The model under review builds one solid part; all positions refer to its coordinate system, in mm. A direction names the side the tool comes from. Round coordinates to 2 decimals unless told otherwise and drop trailing zeros. Order: outer loops, then holes, each group sorted by start corner. A loop starts at its lowest first (then second) coordinate and runs counter-clockwise, first axis right, second up. Notation, with made-up numbers: M 25,-5.5 L 41,-5.5 A9 cw 41,5.5 Z; hole C -28.75,6.5 d10. An arc over 180 degrees is marked long. Answer as a JSON object with one key per item and string values. Group by question number.
1. Mouldability with a two-part tool opening along X and no side actions: class faces 1 (the face through (454.06, -0.04, 521.2)), 2 (the face through (914.4, 0, 1002)), 3 (the face through (0, 0, 1002)), 4 (the face through (451, 0, 0)) as released by +X, released by -X, zero draft, split by the parting line, or undercut.
2. Add section B-B on z = 642. State the section outline as (x, y) points (3 decimals).
3. To check wall thickness, follow probe 1 along Z at (x, y) = (260.5, -4); probe 2 along X at (y, z) = (9, 579); probe 3 along Z at (x, y) = (315, 10) (1 decimal). State the ranges of each line that lie inside material, in increasing order. Write a range as [from, to].
4. Clearance check with flat-ended pins moving along their axes: P1, Ø3, axis at y = -12.5, z = 993, coming from the -X side; P2, Ø4, axis at x = 579, z = 665.5, coming from the -Y side (3 decimals); P3, Ø6, axis at x = 260, z = 1415, coming from the +Y side (3 decimals). State where each tip first meets the part, or that it passes through.
5. Machinability: for faces 5 (the face through (453, 3.175, 1441)), 6 (the face through (44, -22.225, 1030)), 7 (the face through (460.344, -0.044, 518.616)), 8 (the face through (453, -3.175, 1441)), 9 (the face through (451, 0, 2032)), which of the approach directions +Z, -Z, +X, -X, +Y, -Y give a long, thin tool a straight path to every point of the face, cutting with its end or side? Answer none if there is none.
6. Add section A-A on x = 215.5. State the section outline as (y, z) points (1 decimal).
```python
from build123d import *

# Parameters (mm, degrees)
F0_W          = 914.4
F0_H          = 2032
F0_W_2        = 609.6
F0_H_2        = 633.4125
F0_H_3        = 890.5875
F1_DEPTH      = 22.225
F1_DEPTH_BACK = 22.225
F2_W          = 609.6
F2_H          = 890.5875
F2_H_2        = 633.4125
F3_DEPTH      = 3.175
F3_DEPTH_BACK = 3.175
F4_SIZE       = 12.7


# Not quite as in the source:
# - a length typed as a fraction of an inch, garbled in the dataset ("3 / 203.2 mm" for 3/8 in), is restored


with BuildPart() as f1:
    # F0 (on Front) → F1 (new body, two sides)
    with BuildSketch(Plane.XZ) as f1_sk:
        with Locations((457.2, 1016)):
            Rectangle(F0_W, F0_H)
        with Locations((457.2, 519.90625)):
            Rectangle(F0_W_2, F0_H_2, mode=Mode.SUBTRACT)
        with Locations((457.2, 1434.30625)):
            Rectangle(F0_W_2, F0_H_3, mode=Mode.SUBTRACT)
    extrude(amount=F1_DEPTH)
    extrude(f1_sk.sketch, amount=-F1_DEPTH_BACK)

    # F2 (on Front) → F3 (join, two sides)
    with BuildSketch(Plane.XZ) as f3_sk:
        with Locations((457.2, 1434.30625)):
            Rectangle(F2_W, F2_H)
        with BuildLine():
            Line((395.6148101771, 1373.3735846555), (514.1566101771, 1499.5861846555))
            ThreePointArc((514.1566101771, 1499.5861846555), (518.6445346555, 1499.7268398229), (518.7851898229, 1495.2389153445))
            Line((518.7851898229, 1495.2389153445), (400.2433898229, 1369.0263153445))
            ThreePointArc((400.2433898229, 1369.0263153445), (395.7554653445, 1368.8856601771), (395.6148101771, 1373.3735846555))
        make_face(mode=Mode.SUBTRACT)
        with BuildLine():
            Line((395.6148101771, 1411.4735846555), (478.3722068767, 1499.5861846555))
            ThreePointArc((478.3722068767, 1499.5861846555), (482.8601313551, 1499.7268398229), (483.0007865224, 1495.2389153445))
            Line((483.0007865224, 1495.2389153445), (400.2433898229, 1407.1263153445))
            ThreePointArc((400.2433898229, 1407.1263153445), (395.7554653445, 1406.9856601771), (395.6148101771, 1411.4735846555))
        make_face(mode=Mode.SUBTRACT)
        with BuildLine():
            Line((431.3992134776, 1373.3735846555), (514.1566101771, 1461.4861846555))
            ThreePointArc((514.1566101771, 1461.4861846555), (518.6445346555, 1461.6268398229), (518.7851898229, 1457.1389153445))
            Line((518.7851898229, 1457.1389153445), (436.0277931233, 1369.0263153445))
            ThreePointArc((436.0277931233, 1369.0263153445), (431.5398686449, 1368.8856601771), (431.3992134776, 1373.3735846555))
        make_face(mode=Mode.SUBTRACT)
        with Locations((457.2, 519.90625)):
            Rectangle(F2_W, F2_H_2)
        with BuildLine():
            Line((395.6148101771, 497.0735846555), (478.3722068767, 585.1861846555))
            ThreePointArc((478.3722068767, 585.1861846555), (482.8601313551, 585.3268398229), (483.0007865224, 580.8389153445))
            Line((483.0007865224, 580.8389153445), (400.2433898229, 492.7263153445))
            ThreePointArc((400.2433898229, 492.7263153445), (395.7554653445, 492.5856601771), (395.6148101771, 497.0735846555))
        make_face(mode=Mode.SUBTRACT)
        with BuildLine():
            Line((395.6148101771, 458.9735846555), (514.1566101771, 585.1861846555))
            ThreePointArc((514.1566101771, 585.1861846555), (518.6445346555, 585.3268398229), (518.7851898229, 580.8389153445))
            Line((518.7851898229, 580.8389153445), (400.2433898229, 454.6263153445))
            ThreePointArc((400.2433898229, 454.6263153445), (395.7554653445, 454.4856601771), (395.6148101771, 458.9735846555))
        make_face(mode=Mode.SUBTRACT)
        with BuildLine():
            Line((431.3992134776, 458.9735846555), (514.1566101771, 547.0861846555))
            ThreePointArc((514.1566101771, 547.0861846555), (518.6445346555, 547.2268398229), (518.7851898229, 542.7389153445))
            Line((518.7851898229, 542.7389153445), (436.0277931233, 454.6263153445))
            ThreePointArc((436.0277931233, 454.6263153445), (431.5398686449, 454.4856601771), (431.3992134776, 458.9735846555))
        make_face(mode=Mode.SUBTRACT)
    extrude(amount=F3_DEPTH)
    extrude(f3_sk.sketch, amount=-F3_DEPTH_BACK)

    # F4
    f4_edges = [f1.edges().sort_by_distance(p)[0] for p in [
        (457.2, -22.225, 1879.6),
        (762, -22.225, 1434.30625),
        (457.2, -22.225, 989.0125),
        (152.4, -22.225, 1434.30625),
        (457.2, -22.225, 836.6125),
        (152.4, -22.225, 519.90625),
        (762, -22.225, 519.90625),
        (457.2, -22.225, 203.2),
        (457.2, 22.225, 836.6125),
        (762, 22.225, 519.90625),
        (152.4, 22.225, 519.90625),
        (457.2, 22.225, 203.2),
        (152.4, 22.225, 1434.30625),
        (457.2, 22.225, 989.0125),
        (762, 22.225, 1434.30625),
        (457.2, 22.225, 1879.6),
    ]]
    chamfer(f4_edges, length=F4_SIZE)


solid = f1.part
```
Recorded:
{
 "1": {"face 1": "undercut", "face 2": "released by +X", "face 3": "released by -X", "face 4": "zero draft"},
 "2": {"outline": "M 0,-22.225 L 139.7,-22.225 L 152.4,-9.525 L 152.4,-3.175 L 762,-3.175 L 762,-9.525 L 774.7,-22.225 L 914.4,-22.225 L 914.4,22.225 L 774.7,22.225 L 762,9.525 L 762,3.175 L 152.4,3.175 L 152.4,9.525 L 139.7,22.225 L 0,22.225 Z"},
 "3": {"probe 1": "z = [0, 203.2], [836.61, 989.01], [1879.6, 2032]", "probe 2": "x = [0, 152.4], [762, 914.4]", "probe 3": "z = [0, 202.7], [837.1, 988.5], [1880.1, 2032]"},
 "4": {"P1": "stops at x = 0", "P2": "stops at y = -3.175", "P3": "stops at y = 3.175"},
 "5": {"face 5": "+Y", "face 6": "+Z, -Z, +X, -X, -Y", "face 7": "+Y, -Y", "face 8": "-Y", "face 9": "+Z, +X, -X, +Y, -Y"},
 "6": {"outline": "M -22.2,0 L 22.2,0 L 22.2,190.5 L 9.5,203.2 L 3.2,203.2 L 3.2,836.6 L 9.5,836.6 L 22.2,849.3 L 22.2,976.3 L 9.5,989 L 3.2,989 L 3.2,1879.6 L 9.5,1879.6 L 22.2,1892.3 L 22.2,2032 L -22.2,2032 L -22.2,1892.3 L -9.5,1879.6 L -3.2,1879.6 L -3.2,989 L -9.5,989 L -22.2,976.3 L -22.2,849.3 L -9.5,836.6 L -3.2,836.6 L -3.2,203.2 L -9.5,203.2 L -22.2,190.5 Z"}
}
